Answer from the drawing. Dimensions are ordinates in mm from the lowest x, y and z of the part. Coordinates: 2 decimals unless noted, no trailing zeros. Loops run counter-clockwise (first coordinate to the right, second up) from the corner with the lowest first, then second, coordinate; pieces in that order, holes last.
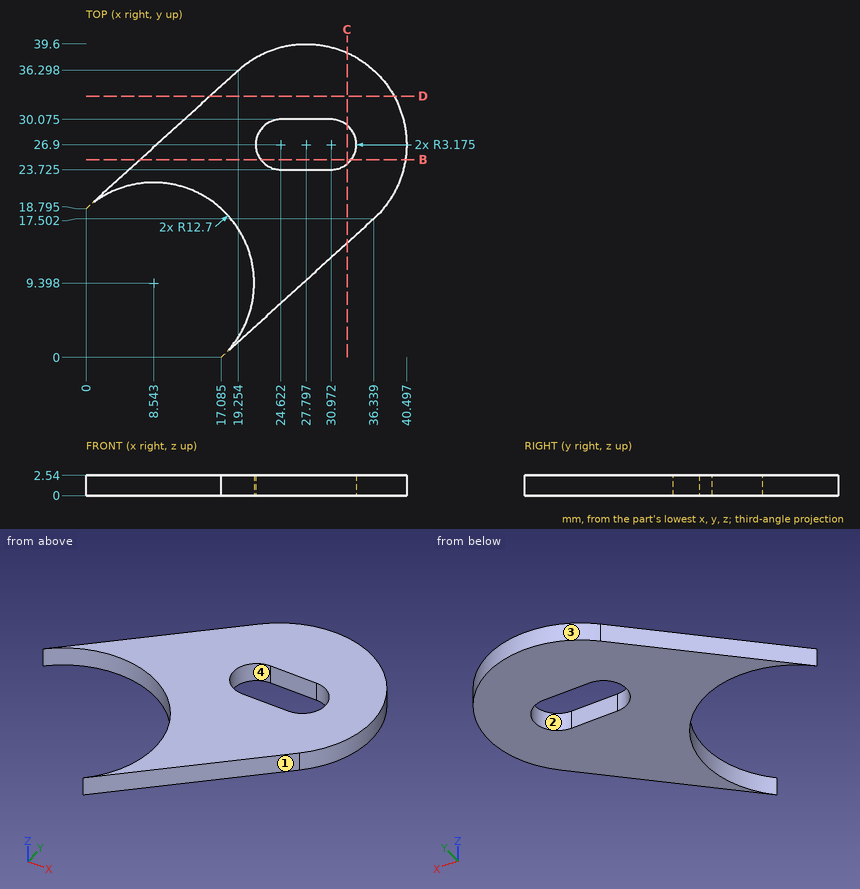
Item 1: A cutting plane is placed at C-C on x = 33. Determine the outline of the cut face in (y, z) (1 decimal), then the cut area to 3 significant figures.
Numbers:
outline: (14.5, 0) - (24.5, 0) - (24.5, 2.5) - (14.5, 2.5) - close; (29.3, 0) - (38.5, 0) - (38.5, 2.5) - (29.3, 2.5) - close
area: 48.6 mm2
Item 2: A cutting plane is placed at B-B on y = 25. Determine the outline of the cut face in (x, z) (1 decimal).
Numbers:
outline: (6.8, 0) - (22.1, 0) - (22.1, 2.5) - (6.8, 2.5) - close; (33.5, 0) - (40.4, 0) - (40.4, 2.5) - (33.5, 2.5) - close
Item 3: A cutting plane is placed at D-D on y = 33. Determine the outline of the cut face in (x, z) (1 decimal).
Numbers:
outline: (15.6, 0) - (38.9, 0) - (38.9, 2.5) - (15.6, 2.5) - close
Item 4: Find the intervals of material crossed by line 1 along Y through (x, z) = (23.5, 1.85); line 2 along Y through (x, z) = (32, 2.1) (1 decimal); line 3 along X through (y, z) = (20.5, 1.7) (1 decimal), in increasing order.
Numbers:
line 1: y = 5.83 to 23.93, 29.87 to 38.85
line 2: y = 13.6 to 23.9, 29.9 to 38.9
line 3: x = 1.9 to 2.4, 14.7 to 38.8
Item 5: Determine the mould class of the marked faces 1, 2, 3 and 4 for opening direction Y: released by +Y, released by -Y, zero draft, split by the parting line, or undercut.
Numbers:
face 1: released by -Y
face 2: undercut
face 3: split by the parting line
face 4: undercut
Item 6: Given pin 1 (1 mm diameter, centred on x = 11.5, z = 1, fed in from +Y) (1 decimal); pin 2 (1.5 mm diameter, centred on x = 6, y = 21, fed in from -Z), each flat-ended and moving along its own axis, determine where each tip first touches the part or whether it passes through.
Numbers:
pin 1: stops at y = 29.7
pin 2: passes through
